Input: part model. Units: mm. Frame: model coordinates. Round coordinates to 2 decimals unless told otherwise and drop trailing zeros. Loops run counter-clockwise (first coordinate to the right, second up) from the corner with the lowest first, then second, coordinate; pieces in that order, holes last. Notation, with made-up numbers: (13, 72.5) - (68, 72.5) arc R29 ccw to (68, 100.5) - close; hole circle Ø2 at (50, 35). An arc over 180 degrees is marked (long way). Write each question's results on one line, items separated by ' | '.
from build123d import *

# Parameters (mm, degrees)
SKETCH_1_R      = 2.1
EXTRUDE_1_DEPTH = 2
FILLET_1_R      = 2


with BuildPart() as part:
    # ｽｹｯﾁ1 → ﾎﾞｽ - 押し出し1 (new body)
    with BuildSketch(Plane.XY):
        Polygon((0, 0), (15, 0), (35, 20), (35, 30), (-20, 30), (-20, 20), align=None)
        with Locations((-15, 25)):
            Circle(SKETCH_1_R, mode=Mode.SUBTRACT)
        with Locations(Location((30, 25, 0), (0, 0, 180))):
            Circle(SKETCH_1_R, mode=Mode.SUBTRACT)
        with Locations((7.5, 25)):
            Circle(SKETCH_1_R, mode=Mode.SUBTRACT)
        with Locations((7.5, 5)):
            Circle(SKETCH_1_R, mode=Mode.SUBTRACT)
    extrude(amount=EXTRUDE_1_DEPTH)

    # ﾌｨﾚｯﾄ1
    fillet_1_edges = [part.edges().sort_by_distance(p)[0] for p in [
        (-20, 20, 1),
        (-20, 30, 1),
        (35, 30, 1),
        (35, 20, 1),
        (15, 0, 1),
        (0, 0, 1),
    ]]
    fillet(fillet_1_edges, radius=FILLET_1_R)


solid = part.part
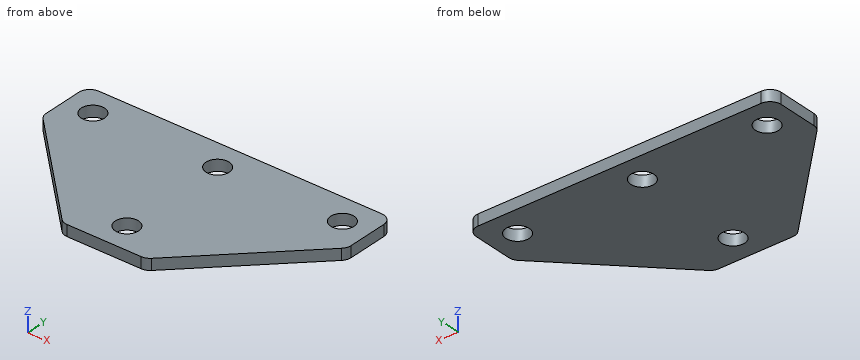
1. Contact query for a flat-ended pin moving along its axis: pin 1 (4 mm diameter, centred on x = 30, y = 25, fed in from +Z). Output: stop coordinate, or through.
Answer:
pin 1: through
2. Section query B-B, the plane y = 5. Output: boundary loops of the cut face in (x, z), plus the area to 3 significant figures.
Answer:
outline: (-5, 0) - (5.4, 0) - (5.4, 2) - (-5, 2) - close; (9.6, 0) - (20, 0) - (20, 2) - (9.6, 2) - close | area: 41.6 mm^2
3. Section query D-D, the plane y = 25. Output: boundary loops of the cut face in (x, z), plus the area to 3 significant figures.
Answer:
outline: (-20, 0) - (-17.1, 0) - (-17.1, 2) - (-20, 2) - close; (-12.9, 0) - (5.4, 0) - (5.4, 2) - (-12.9, 2) - close; (9.6, 0) - (27.9, 0) - (27.9, 2) - (9.6, 2) - close; (32.1, 0) - (35, 0) - (35, 2) - (32.1, 2) - close | area: 84.8 mm^2
4. Line query: line 1 (Y direction, x = 7.5, z = 0.75); line 2 (Y direction, x = 9, z = 1.45); line 3 (Y direction, x = -15, z = 1.4). Output: solid intervals per line, ascending. Write a range as [from, to].
Answer:
line 1: [0, 2.9], [7.1, 22.9], [27.1, 30] | line 2: [0, 3.53], [6.47, 23.53], [26.47, 30] | line 3: [15, 22.9], [27.1, 30]
5. Section query C-C, the plane x = 7.5. Output: boundary loops of the cut face in (y, z).
Answer:
outline: (0, 0) - (2.9, 0) - (2.9, 2) - (0, 2) - close; (7.1, 0) - (22.9, 0) - (22.9, 2) - (7.1, 2) - close; (27.1, 0) - (30, 0) - (30, 2) - (27.1, 2) - close
6. Section query A-A, the plane x = -15. Output: boundary loops of the cut face in (y, z), plus the area to 3 significant figures.
Answer:
outline: (15, 0) - (22.9, 0) - (22.9, 2) - (15, 2) - close; (27.1, 0) - (30, 0) - (30, 2) - (27.1, 2) - close | area: 21.6 mm^2
